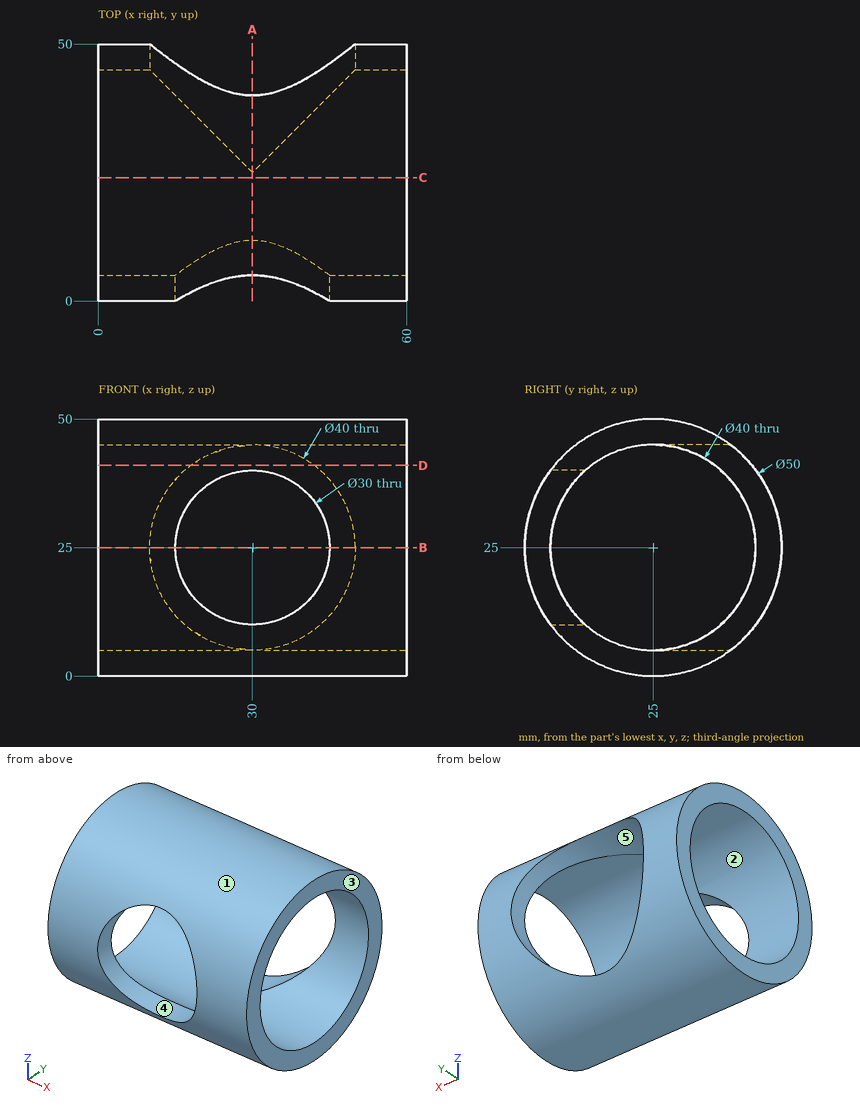
Source: three-view drawing plus pictorial views. Frame: mm from the lowest corner of the part. A direction names the side the tool comes from. Round coordinates to 2 decimals unless told otherwise and drop trailing zeros. Loops run counter-clockwise (first coordinate to the right, second up) from the corner with the lowest first, then second, coordinate; pieces in that order, holes last. Notation, with made-up numbers: M 60,11.5 L 73,11.5 A8 ccw 73,22.5 Z; hole C 4.5,22.25 d2. An arc over 180 degrees is marked long. Answer as CSV lines item,"result". Start each with the question number.
(1) Section C-C, the plane y = 24. Output: boundary loops of the cut face in (x, z), plus the area to 3 significant figures.
(2) Section A-A, the plane x = 30. Output: boundary loops of the cut face in (y, z), plus the area to 3 significant figures.
(3) First-contact query: pin 1 (1 mm diameter, centred on x = 30.5, y = 26.5, fed in from +Z); pin 2 (6 mm diameter, centred on x = 29, y = 23.5, fed in from -Z); pin 3 (2 mm diameter, centred on x = 32, y = 38, fed in from +Z); pin 4 (10 mm diameter, centred on x = 51.5, z = 16.5, fed in from -Y). Flat tips, straight axial feed; report the tip coordinate or a pass-through.
(4) Reachability of the marked faces 4 and 5 from +Z, -Z, +X, -X, +Y, -Y: full face, straight path, thin tool, end or side. Return the list, or none.
(5) Draft query along Y for the marked faces 1, 2 and 3. Return one class per face: released by +Y, released by -Y, zero draft, split by the parting line, or undercut.
(6) Section B-B, the plane z = 25. Output: boundary loops of the cut face in (x, y).
(7) Line query: line 1 (X direction, y = 3.25, z = 25); line 2 (Y direction, x = 10, z = 39); line 3 (Z direction, x = 28, y = 27). Output: solid intervals per line, ascending. Write a range as [from, to].
(8) Section D-D, the plane z = 41. Output: boundary loops of the cut face in (x, y).
Values found:
1,outline,"M 0,0.02 L 60,0.02 L 60,5.03 L 0,5.03 Z; M 0,44.97 L 60,44.97 L 60,49.98 L 0,49.98 Z"
1,area,"601 mm²"
2,outline,"M 5,10 A25 ccw 40,5 L 25,5 A20 cw 11.77,10 Z; M 5,40 L 11.77,40 A20 cw 25,45 L 40,45 A25 ccw Z"
2,area,"291 mm²"
3,pin 1,"stops at z = 49.98"
3,pin 2,"stops at z = 0"
3,pin 3,"stops at z = 46.93"
3,pin 4,"stops at y = 0.25"
4,face 4,"+Y, -Y"
4,face 5,"+Y"
5,face 1,"split by the parting line"
5,face 2,"undercut"
5,face 3,"zero draft"
6,outline,"M 0,0 L 15,0 L 15,5 L 0,5 Z; M 0,45 L 10,45 L 10,50 L 0,50 Z; M 45,0 L 60,0 L 60,5 L 45,5 Z; M 50,45 L 60,45 L 60,50 L 50,50 Z"
7,line 1,"x = [0, 15], [45, 60]"
7,line 2,"y = [4.29, 10.72], [39.28, 45.71]"
7,line 3,"z = [0.08, 5.1], [44.9, 49.92]"
8,outline,"M 0,5.79 L 60,5.79 L 60,13 L 0,13 Z; M 0,37 L 18,37 L 18,44.21 L 0,44.21 Z; M 42,37 L 60,37 L 60,44.21 L 42,44.21 Z"
